```python
from build123d import *

# Parameters (mm, degrees)
BOSS_EXTRUDE1_DEPTH = 5.08
SKETCH2_W           = 101.6
SKETCH2_H           = 10.16
CUT_EXTRUDE3_DEPTH  = 22.86
SKETCH9_R           = 1.27
CUT_EXTRUDE4_DEPTH  = 25.908
SKETCH13_W          = 11.0236
SKETCH13_H          = 5.0038
CUT_EXTRUDE5_DEPTH  = 25.908
SKETCH8_R           = 8.636
CUT_EXTRUDE6_DEPTH  = 25.908
SKETCH14_W          = 212.203069611
SKETCH14_H          = 122.52066239
SKETCH14_W_2        = 52.5744
SKETCH14_H_2        = 29.137232508
CUT_EXTRUDE7_DEPTH  = 25.908
SKETCH15_W          = 52.5744
SKETCH15_H          = 43.722211583
BOSS_EXTRUDE2_DEPTH = 5.08
SKETCH17_W          = 25.579382718
SKETCH17_H          = 36.902767492
CUT_EXTRUDE8_DEPTH  = 10.16
SKETCH18_R          = 1.7526
CUT_EXTRUDE9_DEPTH  = 10.16


with BuildPart() as part:
    # Sketch1 → Boss-Extrude1 (new body)
    with BuildSketch(Plane(origin=(0, 0, 0), x_dir=(0, 0, -1), z_dir=(1, 0, 0))):
        Polygon((62.997029703, -55.82970297), (88.397029703, -55.82970297), (88.397029703, -65.98970297), (-89.402970297, -65.98970297), (-89.402970297, -55.82970297), (-64.002970297, -55.82970297), (-64.002970297, 27.837475742), (62.997029703, 27.837475742), align=None)
    extrude(amount=BOSS_EXTRUDE1_DEPTH)

    # Sketch2 → Cut-Extrude3 (cut)
    with BuildSketch(Plane(origin=(0, 0, 0), x_dir=(0, 0, -1), z_dir=(1, 0, 0))):
        with Locations((-0.502970297, -60.90970297)):
            Rectangle(SKETCH2_W, SKETCH2_H)
    extrude(amount=CUT_EXTRUDE3_DEPTH, mode=Mode.SUBTRACT)

    # Sketch9 → Cut-Extrude4 (cut)
    with BuildSketch(Plane(origin=(0, 0, 0), x_dir=(0, 0, -1), z_dir=(1, 0, 0))):
        with Locations((-22.010170297, -1.223907747)):
            Circle(SKETCH9_R)
        with Locations(Location((-22.010170297, -18.977232508, 0), (0, 0, 180))):
            Circle(SKETCH9_R)
        with Locations((20.404229703, -18.977232508)):
            Circle(SKETCH9_R)
        with Locations(Location((20.404229703, -1.223907747, 0), (0, 0, 180))):
            Circle(SKETCH9_R)
    extrude(amount=CUT_EXTRUDE4_DEPTH, mode=Mode.SUBTRACT)

    # Sketch13 → Cut-Extrude5 (cut)
    with BuildSketch(Plane(origin=(0, 0, 0), x_dir=(0, 0, -1), z_dir=(1, 0, 0))):
        with Locations((-0.746414126, -2.5019)):
            Rectangle(SKETCH13_W, SKETCH13_H)
    extrude(amount=CUT_EXTRUDE5_DEPTH, mode=Mode.SUBTRACT)

    # Sketch8 → Cut-Extrude6 (cut)
    with BuildSketch(Plane(origin=(0, 0, 0), x_dir=(0, 0, -1), z_dir=(1, 0, 0))):
        with Locations((12.197029703, -10.100570128)):
            Circle(SKETCH8_R)
        with Locations((-13.710970297, -10.100570128)):
            Circle(SKETCH8_R)
    extrude(amount=CUT_EXTRUDE6_DEPTH, mode=Mode.SUBTRACT)

    # Sketch14 → Cut-Extrude7 (cut)
    with BuildSketch(Plane(origin=(0, 0, 0), x_dir=(0, 0, -1), z_dir=(1, 0, 0))):
        with Locations((-5.581398167, -16.698007888)):
            Rectangle(SKETCH14_W, SKETCH14_H)
        with Locations((-0.802970297, -9.488616254)):
            Rectangle(SKETCH14_W_2, SKETCH14_H_2, mode=Mode.SUBTRACT)
    extrude(amount=CUT_EXTRUDE7_DEPTH, mode=Mode.SUBTRACT)

    # Sketch15 → Boss-Extrude2 (add)
    with BuildSketch(Plane(origin=(0, 0, 0), x_dir=(0, 0, -1), z_dir=(1, 0, 0))):
        with Locations((-0.802970297, -44.178894209)):
            Rectangle(SKETCH15_W, SKETCH15_H)
    extrude(amount=BOSS_EXTRUDE2_DEPTH)

    # Sketch17 → Cut-Extrude8 (cut)
    with BuildSketch(Plane(origin=(0, 0, 0), x_dir=(0, 0, -1), z_dir=(1, 0, 0))):
        with Locations((-17.869691359, -42.508616254)):
            Rectangle(SKETCH17_W, SKETCH17_H)
        with Locations((17.869691359, -42.508616254)):
            Rectangle(SKETCH17_W, SKETCH17_H)
    extrude(amount=CUT_EXTRUDE8_DEPTH, mode=Mode.SUBTRACT)

    # Sketch18 → Cut-Extrude9 (cut)
    with BuildSketch(Plane(origin=(0, -66.04, 0), x_dir=(1, 0, 0), z_dir=(0, 1, 0))):
        with Locations(Location((2.54, -22.010170297, 0), (0, 0, 270))):
            Circle(SKETCH18_R)
        with Locations(Location((2.54, 20.404229703, 0), (0, 0, 90))):
            Circle(SKETCH18_R)
    extrude(amount=CUT_EXTRUDE9_DEPTH, mode=Mode.SUBTRACT)


solid = part.part
```
Model file for the job. Use its own axes, mm. A direction names the side the tool comes from. Give positions to 0.01 mm unless a question says otherwise; leave off trailing zeros. Loops run counter-clockwise (first coordinate to the right, second up) from the corner with the lowest first, then second, coordinate; pieces in that order, holes last. Notation, with made-up numbers: (50, 11) -> (98, 11) arc R16 ccw to (98, 19) -> close; hole circle Ø2 at (-7.5, 21.25). An arc over 180 degrees is marked (long way). Use CSV: the item, a comma, the result in double quotes. Start each with the question number.
1) Slice it at B-B on x = 2.54. Give the number of separate pieces and of enclosed holes in the cut face, plus the area to 3 significant figures.
2) Mould opens along Y. For faces 6 (the flat face through (3, 5.08, 1)), 7 (the flat face through (5.08, -30, 1)), 8 (the flat face through (3, -24.057, -15)) say: released by +Y, released by -Y, zero draft, split by the parting line, or undercut.
3) Slice it at A-A on z = -2.5. Give the cut face in (x, y).
4) Slice it at C-C on z = 17.5. Give the cut face in (x, y).
5) Flat gauge pins, fed straight in: pin 1 Ø2.5 at (x, y) = (1.5, -39.5) entering from +Z; pin 2 Ø15.5 at (y, z) = (-10.1, 13.71) entering from -X; pin 3 Ø1.5 at (x, y) = (2, -41.5) entering from -Z. Where does each tip first touch, or does it go through?
6) Slice it at D-D on y = -42.5. Give the cut face in (x, z), plus the area to 3 significant figures.
7) Tool access for faces 1 (the flat face through (3, 0, 1)), 2 (the flat face through (0, -30, 1)), 3 (the flat face through (3, -60.96, 16)), 4 (the flat face through (3, -66.04, 1)), 5 (the cylindrical face through (2.014, -63.536, -22.076)): list every direction of +Z, -Z, +X, -X, +Y, -Y with a clear straight run to the whole face (end or side of a thin tool).
8) Wall check: line 1 (Y direction, x = 1.8, z = -12.5); line 2 (Y direction, x = 1.8, z = -0.5); line 3 (Z direction, x = 0.4, y = -1). Give the ranges that are in metal, low to high.
Computed values:
1,separate pieces,"3"
1,enclosed holes,"7"
1,area,"1,590 mm^2"
2,face 6,"released by +Y"
2,face 7,"zero draft"
2,face 8,"undercut"
3,outline,"(0, -66.04) -> (5.08, -66.04) -> (5.08, -5) -> (0, -5) -> close; (0, 0) -> (5.08, 0) -> (5.08, 5.08) -> (0, 5.08) -> close"
4,outline,"(0, -66.04) -> (5.08, -66.04) -> (5.08, -60.96) -> (0, -60.96) -> close; (0, -24.06) -> (5.08, -24.06) -> (5.08, -17.86) -> (0, -17.86) -> close; (0, -2.34) -> (5.08, -2.34) -> (5.08, 5.08) -> (0, 5.08) -> close"
5,pin 1,"stops at z = 5.08"
5,pin 2,"passes through"
5,pin 3,"stops at z = -5.08"
6,outline,"(0, -5.08) -> (5.08, -5.08) -> (5.08, 5.08) -> (0, 5.08) -> close"
6,area,"51.6 mm^2"
7,face 1,"+X, -X"
7,face 2,"+Z, -Z, -X, +Y, -Y"
7,face 3,"+Z, +X, -X"
7,face 4,"+Z, -Z, +X, -X, -Y"
7,face 5,"-Y"
8,line 1,"y = -66.04 to -60.96, -24.06 to -18.73, -1.47 to 5.08"
8,line 2,"y = -66.04 to -5, 0 to 5.08"
8,line 3,"z = -25.48 to -21.65, -19.15 to -4.77, 6.26 to 20.76, 23.26 to 27.09"
